Autodesk Inventor part; units mm, degrees
ref_plane "YZ Plane" through (0, 0, 0) normal (1, 0, 0) x (0, 1, 0)
ref_plane "XZ Plane" through (0, 0, 0) normal (0, 1, 0) x (-1, 0, 0)
ref_plane "XY Plane" through (0, 0, 0) normal (0, 0, 1) x (1, 0, 0)
sketch "Sketch1" plane through (0, 0, 0) normal (0, 1, 0) x (-1, 0, 0)
  line L0 (7.5264, 21.8341) -> (7.5264, 13.5841)
  line L1 (7.5264, 13.5841) -> (1.7974, 7.6477)
  line L2 (1.7974, 7.6477) -> (-6.4526, 7.6477)
  line L3 (7.5264, 21.8341) -> (1.6928, 27.6678)
  line L4 (1.6928, 27.6678) -> (-6.5572, 27.6678)
  line L5 (-6.5572, 27.6678) -> (-12.2862, 21.7314)
  line L6 (-12.2862, 21.7314) -> (-12.2862, 13.4814)
  line L7 (-12.2862, 13.4814) -> (-6.4526, 7.6477)
  line L8 (9.9412, 22.8339) -> (9.9412, 12.5839)
  line L9 (9.9412, 12.5839) -> (2.7976, 5.2333)
  line L10 (2.7976, 5.2333) -> (-7.4524, 5.2333)
  line L11 (9.9412, 22.8339) -> (2.6934, 30.0818)
  line L12 (2.6934, 30.0818) -> (-7.5566, 30.0818)
  line L13 (-7.5566, 30.0818) -> (-14.7002, 22.7311)
  line L14 (-14.7002, 22.7311) -> (-14.7002, 12.4811)
  line L15 (-14.7002, 12.4811) -> (-7.4524, 5.2333)
  point P0 (0, 0)
  point P1 (1, 1)
  dimension "d0" = 8.25
  dimension "d3" = 8.25
  dimension "d5" = 8.25
  dimension "d7" = 8.25
  dimension "d8" = 8.25
  dimension "d9" = 8.25
  dimension "d12" = 8.25
  dimension "d17" = 8.25
  dimension "d18" = 135
  dimension "d19" = 10.25
  dimension "d20" = 10.25
  dimension "d21" = 10.25
  dimension "d22" = 10.25
  dimension "d23" = 10.25
  dimension "d24" = 10.25
  dimension "d25" = 10.25
  dimension "d26" = 10.25
  dimension "d27" = 135
  dimension "d29" = 2.414
  dimension "d31" = 2.414
  dimension "d32" = 2.4144
  dimension "d33" = 2.4148
extrude "OutsideHeight" add sketch "Sketch1" along normal blind 10
extrude "BaseHeight" add sketch "Sketch1" along normal blind 1 contours L0 L1 L2 L7 L6 L5 L4 L3
sketch "Sketch2" plane through (-2.6934, 0, 30.0818) normal (-0.7071, 0, 0.7071) x (0.7071, 0, 0.7071)
  line L0 (-10.25, 10) -> (0, 10)
  line L1 (-0.1464, 0) -> (-10.3964, 0)
  line L2 (-8.75, 10) -> (-1.5, 10)
  line L3 (-10.25, 0) -> (-10.25, 10)
  line L4 (0, 0) -> (0, 10)
  line L5 (-8.75, 1) -> (-1.5, 1)
  line L6 (-8.75, 10) -> (-8.75, 1)
  line L7 (-1.5, 10) -> (-1.5, 1)
  point P0 (-19.3665, 0)
  dimension "d41" = 1.5
  dimension "d42" = 1.5
  dimension "d43" = 1
extrude "SideCut" cut sketch "Sketch2" against normal blind 2.5
equation "\"d3\" = d0"
equation "\"d5\" = d0"
equation "\"d7\" = d0"
equation "\"d8\" = d0"
equation "\"d9\" = d0"
equation "\"d12\" = d0"
equation "\"d17\" = d0"
equation "\"d20\" = d19"
equation "\"d21\" = d19"
equation "\"d22\" = d19"
equation "\"d23\" = d19"
equation "\"d24\" = d19"
equation "\"d25\" = d19"
equation "\"d26\" = d19"
equation "\"d42\" = d41"
properties part number "TokenHolderSingle"
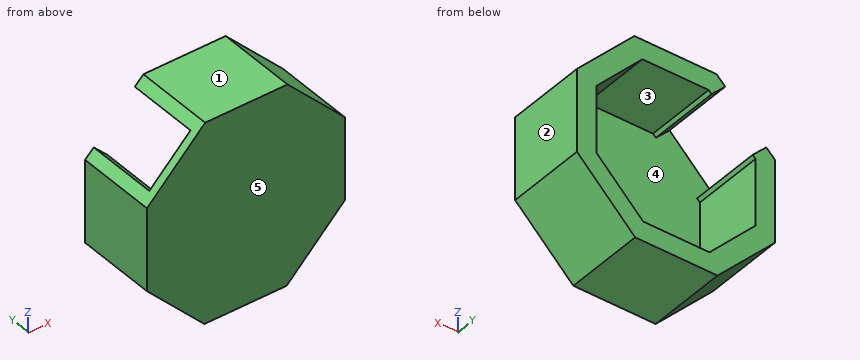
Work out the finished part from the listing and answer in its coordinate system (mm). Face numbers are marked on the shaded views. A direction names the side the tool comes from. Round coordinates to 2 decimals unless told otherwise and drop trailing zeros. Write each loop counter-clockwise with the first axis right and the second up, starting at its lowest first coordinate (ties: lowest second). Pieces come first, ordered by that corner, then holes.
1) A cutting plane is placed at D-D on z = 26.5. Determine the outline of the cut face in (x, y), and give its area (3 significant figures).
2) Consider probe 1 along X at (y, z) = (1.75, 14.5); probe 2 along Z at (x, y) = (4.75, 3.75); probe 3 along Y at (x, z) = (8.5, 24). Determine where each line is inside the solid, lowest interval first.
3) Determine the mould class of the marked faces 1, 2 and 3 for opening direction X: pulls with the +X half, pulls with the -X half, needs draft (parallel to the pull), parting line crosses it, or undercut.
4) Which of the six approach directions +Z, -Z, +X, -X, +Y, -Y give full straight-line access (tool end or side, diameter ignored) to the marked faces 4 and 5?
5) A flat-ended cylindrical pin translates along its axis: P1, Ø3, axis at x = -2, z = 19.5, coming from the +Y side. Find the tip coordinate at first contact, or state that the pin passes through.
6) A cutting plane is placed at B-B on z = 20.25. Determine the outline of the cut face in (x, y), and give its area (3 significant figures).
7) A cutting plane is placed at C-C on x = 8. Determine the outline of the cut face in (y, z), and give its area (3 significant figures).
8) A cutting plane is placed at A-A on y = 5.5. Determine the outline of the cut face in (x, z).
Entries:
1. outline: (-6.28, 0) - (11.04, 0) - (11.04, 10) - (7.68, 10) - (7.68, 1) - (-6.28, 1) - close
1. area: 47.5 mm2
2. probe 1: x = -9.94 to -7.53, 12.29 to 14.7
2. probe 2: z = 5.23 to 7.65, 27.67 to 30.08
2. probe 3: y = 0 to 1
3. face 1: needs draft
3. face 2: pulls with the +X half
3. face 3: undercut
4. face 4: +Y
4. face 5: +Z, -Z, +X, -X, -Y
5. P1: stops at y = 1
6. outline: (-9.94, 0) - (14.7, 0) - (14.7, 10) - (12.29, 10) - (12.29, 1) - (-7.53, 1) - (-7.53, 10) - (-9.94, 10) - close
6. area: 68.1 mm2
7. outline: (0, 5.78) - (10, 5.78) - (10, 9.2) - (1, 9.2) - (1, 26.17) - (10, 26.17) - (10, 29.63) - (0, 29.63) - close
7. area: 85.6 mm2
8. outline: (-9.94, 12.58) - (-2.8, 5.23) - (7.45, 5.23) - (14.7, 12.48) - (14.7, 22.73) - (7.56, 30.08) - (-2.69, 30.08) - (-3.75, 29.02) - (-2.05, 27.31) - (-1.69, 27.67) - (6.56, 27.67) - (12.29, 21.73) - (12.29, 13.48) - (6.45, 7.65) - (-1.8, 7.65) - (-7.53, 13.58) - (-7.53, 21.83) - (-7.17, 22.19) - (-8.88, 23.89) - (-9.94, 22.83) - close
